Model file for the job. Use its own axes, mm. Face numbers are marked on the shaded views. Give positions to 0.01 mm unless a question says otherwise; leave off trailing zeros. Write each loop counter-clockwise with the first axis right and the second up, starting at its lowest first coordinate (ties: lowest second). Pieces come first, ordered by that corner, then holes.
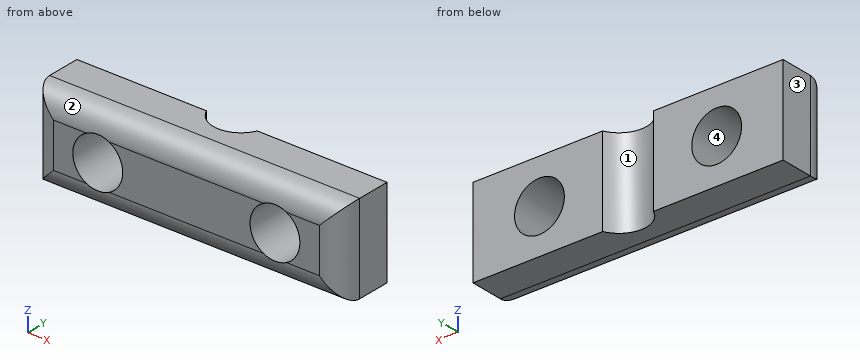
```python
from build123d import *

# Parameters (mm, degrees)
SKETCH1_W           = 28
SKETCH1_H           = 8
SKETCH1_R           = 2.25
BOSS_EXTRUDE1_DEPTH = 5
CUT_EXTRUDE1_REACH  = 31.547
FILLET1_R           = 2


with BuildPart() as part:
    # Sketch1 → Boss-Extrude1 (new body)
    with BuildSketch(Plane(origin=(0, 0, 0), x_dir=(1, 0, 0), z_dir=(0, 1, 0))):
        with Locations((14, 4)):
            Rectangle(SKETCH1_W, SKETCH1_H)
        with Locations(Location((6, 4, 0), (0, 0, 270))):
            Circle(SKETCH1_R, mode=Mode.SUBTRACT)
        with Locations(Location((22, 4, 0), (0, 0, 270))):
            Circle(SKETCH1_R, mode=Mode.SUBTRACT)
    extrude(amount=BOSS_EXTRUDE1_DEPTH)

    # Sketch2 → Cut-Extrude1 (cut, up to next)
    with BuildSketch(Plane.XY, mode=Mode.PRIVATE) as cut_extrude1_sk1:
        with BuildLine():
            Line((11.5, 6), (16.5, 6))
            ThreePointArc((16.5, 6), (14, 3.5), (11.5, 6))
        make_face()
    cut_extrude1_tool1 = extrude(cut_extrude1_sk1.sketch, amount=-CUT_EXTRUDE1_REACH, mode=Mode.PRIVATE) & part.part
    add(cut_extrude1_tool1.solids().sort_by_distance((14, 4.938967, 0))[0], mode=Mode.SUBTRACT)

    # Fillet1
    # the kernel refuses this fillet: 2 mm, written as the material it takes off along each edge
    with BuildSketch(Plane(origin=(-5, 0, -8), x_dir=(0, 1, 0), z_dir=(1, 0, 0))) as fillet1_piece_1:
        with BuildLine():
            CenterArc((FILLET1_R, FILLET1_R), FILLET1_R, 180, 90)
            Line((0, FILLET1_R), (0, 0))
            Line((0, 0), (FILLET1_R, 0))
        make_face()
    extrude(amount=38, mode=Mode.SUBTRACT)
    with BuildSketch(Plane(origin=(28, 0, -13), x_dir=(-1, 0, 0), z_dir=(0, 0, 1)), Plane(origin=(0, 0, 5), x_dir=(1, 0, 0), z_dir=(0, 0, -1))) as fillet1_piece_2:
        with BuildLine():
            CenterArc((FILLET1_R, -FILLET1_R), FILLET1_R, 90, 90)
            Line((0, -FILLET1_R), (0, 0))
            Line((0, 0), (FILLET1_R, 0))
        make_face()
    extrude(amount=18, mode=Mode.SUBTRACT)
    with BuildSketch(Plane(origin=(33, 0, 0), x_dir=(0, 0, -1), z_dir=(-1, 0, 0))) as fillet1_piece_3:
        with BuildLine():
            CenterArc((FILLET1_R, -FILLET1_R), FILLET1_R, 90, 90)
            Line((0, -FILLET1_R), (0, 0))
            Line((0, 0), (FILLET1_R, 0))
        make_face()
    extrude(amount=38, mode=Mode.SUBTRACT)


solid = part.part
```
1. Slice it at B-B, the plane z = -4. Write the cut outline in (x, y), and give its area (3 significant figures).
Calculated:
outline: (0, 2) arc R2 ccw to (2, 0) - (3.75, 0) - (3.75, 5) - (0, 5) - close; (8.25, 0) - (19.75, 0) - (19.75, 5) - (16.29, 5) arc R2.5 cw to (11.71, 5) - (8.25, 5) - close; (24.25, 0) - (26, 0) arc R2 ccw to (28, 2) - (28, 5) - (24.25, 5) - close
area: 88.3 mm2
2. Slice it at D-D, the plane x = 2.5. Write the cut outline in (y, z), and give its area (3 significant figures).
Calculated:
outline: (0, -6) arc R2 ccw to (2, -8) - (5, -8) - (5, 0) - (2, 0) arc R2 ccw to (0, -2) - close
area: 38.3 mm2
3. Probe probe 1 along X at (y, z) = (2.45, -4); probe 2 along X at (y, z) = (4.6, -4.5); probe 3 along Z at (x, y) = (6, 3.5). List the from-to ranges inside material, lowest first.
Calculated:
probe 1: x = 0 to 3.75, 8.25 to 19.75, 24.25 to 28
probe 2: x = 0 to 3.81, 8.19 to 11.93, 16.07 to 19.81, 24.19 to 28
probe 3: z = -8 to -6.25, -1.75 to 0
4. Pull direction X, two halves, no side cores. Call the marked faces 1, 2, 3 and 4: +X half, -X half, draft (parallel to the pull), parting line (faces both ways), or undercut.
Calculated:
face 1: undercut
face 2: draft
face 3: -X half
face 4: undercut
5. Slice it at C-C, the plane x = 6. Write the cut outline in (y, z), and give its area (3 significant figures).
Calculated:
outline: (0.02, -6.25) arc R2 ccw to (2, -8) - (5, -8) - (5, -6.25) - close; (0.02, -1.75) - (5, -1.75) - (5, 0) - (2, 0) arc R2 ccw to start
area: 15.8 mm2
6. Pin check, flat tip, straight feed: P1, Ø1.5, axis at x = 7.5, y = 1, coming from the +Z side. Stop position of the tip, or through.
Calculated:
P1: stops at z = -0.02
7. Slice it at A-A, the plane y = 4.45. Write the cut outline in (x, z), and give its area (3 significant figures).
Calculated:
outline: (0, -8) - (12.04, -8) - (12.04, 0) - (0, 0) - close; (15.96, -8) - (28, -8) - (28, 0) - (15.96, 0) - close; hole circle Ø4.5 at (6, -4); hole circle Ø4.5 at (22, -4)
area: 161 mm2
